Verification items for this drawing (mm, ordinates from the low corner). A direction names the side the tool comes from. Round coordinates to 2 decimals unless told otherwise and drop trailing zeros. Order: outer loops, then holes, each group sorted by start corner. A loop starts at its lowest first (then second) coordinate and runs counter-clockwise, first axis right, second up. Notation, with made-up numbers: (-13.5, -9) - (28.5, -9) arc R25 cw to (28.5, 24) - close; hole circle Ø1 at (26.5, -25). An arc over 180 degrees is marked (long way). Use a Markdown table: item, result. Add a question column.
(1) Mould release check, pull along Y, two halves, no side actions. Record for the marked faces 3, 4 and 5: released by +Y, released by -Y, zero draft, split by the parting line, or undercut.
(2) Section check A-A on y = 5.5. Record the boundary of the cut face in (x, z), then the cut area to 3 significant figures.
(3) Access from +Z, -Z, +X, -X, +Y, -Y to the whole of each face (thin tool, end or side, straight path). Record for the marked faces 1 and 2.
(4) Section check C-C on z = 0.5. Record the boundary of the cut face in (x, y), then the cut area to 3 significant figures.
(5) Gauge pin test, flat end, axial feed: P1, Ø1.2, axis at x = 11, z = 2.5, coming from the -Y side. Record the tip position at first contact, or that the pin passes through.
(6) Thickness scan on line 1 along X through (y, z) = (12.25, 2.15); line 2 along Y through (x, z) = (10.25, 0.2). Record the ranges inside material, lowest first. Write a range as [from, to].
(7) Section check B-B on x = 5. Record the boundary of the cut face in (y, z).
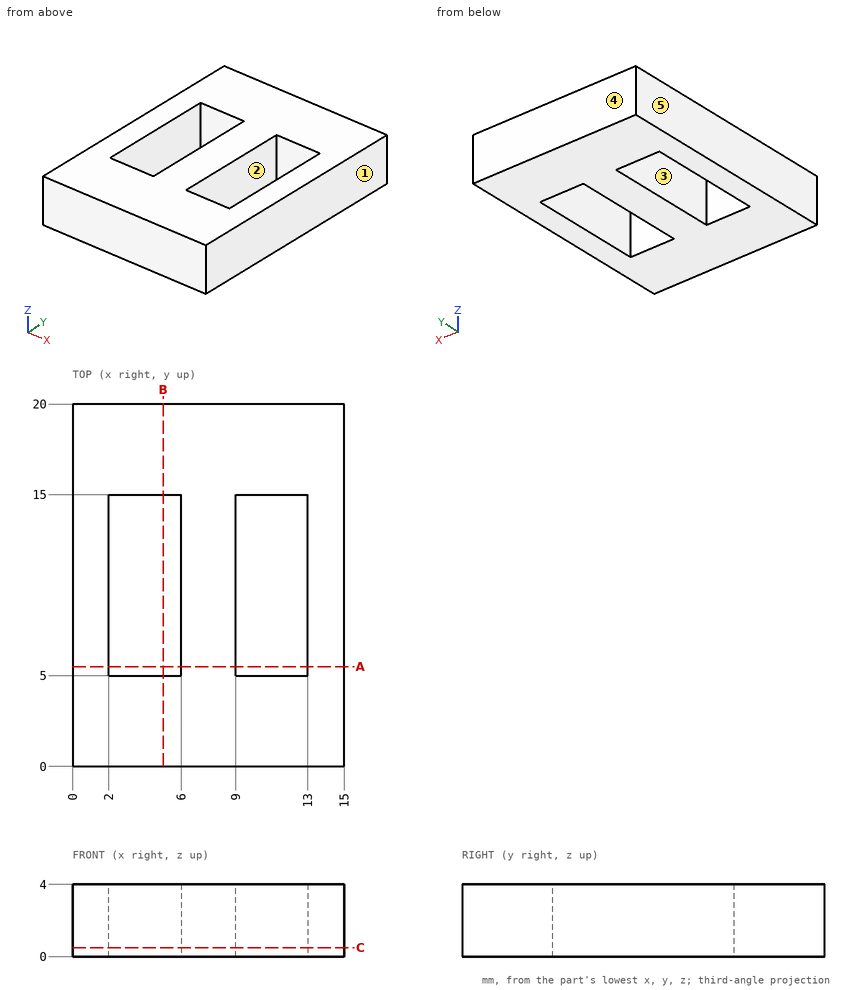
Check sheet entries:
| question | item | result |
|---|---|---|
| 1 | face 3 | undercut |
| 1 | face 4 | released by +Y |
| 1 | face 5 | zero draft |
| 2 | outline | (0, 0) - (2, 0) - (2, 4) - (0, 4) - close; (6, 0) - (9, 0) - (9, 4) - (6, 4) - close; (13, 0) - (15, 0) - (15, 4) - (13, 4) - close |
| 2 | area | 28.0 mm2 |
| 3 | face 1 | +Z, -Z, +X, +Y, -Y |
| 3 | face 2 | +Z, -Z |
| 4 | outline | (0, 0) - (15, 0) - (15, 20) - (0, 20) - close; hole (2, 5) - (6, 5) - (6, 15) - (2, 15) - close; hole (9, 5) - (13, 5) - (13, 15) - (9, 15) - close |
| 4 | area | 220 mm2 |
| 5 | P1 | stops at y = 0 |
| 6 | line 1 | x = [0, 2], [6, 9], [13, 15] |
| 6 | line 2 | y = [0, 5], [15, 20] |
| 7 | outline | (0, 0) - (5, 0) - (5, 4) - (0, 4) - close; (15, 0) - (20, 0) - (20, 4) - (15, 4) - close |
